Could you check a few things on this model? Use its own coordinates, in mm. A direction names the side the tool comes from. Round coordinates to 2 decimals unless told otherwise and drop trailing zeros. Loops run counter-clockwise (first coordinate to the right, second up) from the corner with the lowest first, then second, coordinate; pieces in that order, holes last. Notation, with made-up numbers: M 28.25,34.5 L 71.25,34.5 A31 ccw 71.25,65.5 Z; hole C 74.5,50.5 d1. An arc over 180 degrees is marked long. Answer in a Markdown table with one row per item.
```python
from build123d import *

# Parameters (mm, degrees)
BOSS_EXTRUDE1_DEPTH = 180.975
FILLET1_R           = 6.35


with BuildPart() as part:
    # Sketch1 → Boss-Extrude1 (new body, symmetric)
    with BuildSketch(Plane(origin=(0, 0, 0), x_dir=(0, 0, -1), z_dir=(1, 0, 0))):
        with BuildLine():
            ThreePointArc((-1.052151583, -0.382951858), (0.017010399, -0.096470768), (1.119676327, 0))
            Line((1.119676327, 0), (138.580323673, 0))
            Line((138.580323673, 0), (138.580323673, 6.35))
            Line((138.580323673, 6.35), (1.119676327, 6.35))
            ThreePointArc((1.119676327, 6.35), (-1.085655529, 6.157058463), (-3.223979493, 5.584096284))
            Line((-3.223979493, 5.584096284), (-72.724254031, -19.711934921))
            Line((-72.724254031, -19.711934921), (-70.552426121, -25.678983063))
            Line((-70.552426121, -25.678983063), (-1.052151583, -0.382951858))
        make_face()
    extrude(amount=BOSS_EXTRUDE1_DEPTH, both=True)

    # Fillet1
    fillet1_edges = [part.edges().sort_by_distance(p)[0] for p in [
        (-180.975, -22.695458992, 71.638340076),
        (180.975, -22.695458992, 71.638340076),
        (180.975, 3.175, -138.580323673),
        (-180.975, 3.175, -138.580323673),
    ]]
    fillet(fillet1_edges, radius=FILLET1_R)


solid = part.part
```
1) I want a section at A-A, the plane x = 95. Please give me the cut outline in (y, z), plus the area to 3 significant figures.
Computed:
| item | result |
|---|---|
| outline | M -25.68,70.55 L -0.38,1.05 A6.35 cw 0,-1.12 L 0,-138.58 L 6.35,-138.58 L 6.35,-1.12 A12.7 ccw 5.58,3.22 L -19.71,72.72 Z |
| area | 1,360 mm² |
2) I want a section at C-C, the plane y = -11. Please give me the cut outline in (x, z) (3 decimals), plus the area to 3 significant figures.
Computed:
| item | result |
|---|---|
| outline | M -180.975,30.222 L 180.975,30.222 L 180.975,48.788 L -180.975,48.788 Z |
| area | 6,720 mm² |
3) I need wall thicknesses on line 1 (Y direction, x = -26.5, z = -65.5); line 2 (Y direction, x = 132, z = 50). Which ranges of each line are inside material? Lowest first, please.
Computed:
| item | result |
|---|---|
| line 1 | y = 0 to 6.35 |
| line 2 | y = -18.2 to -11.44 |
4) I want a section at B-B, the plane z = -58. Please give me the cut outline in (x, y) (3 decimals), plus the area to 3 significant figures.
Computed:
| item | result |
|---|---|
| outline | M -180.975,0 L 180.975,0 L 180.975,6.35 L -180.975,6.35 Z |
| area | 2,300 mm² |
5) Which directions (+Z, -Z, +X, -X, +Y, -Y) give clear straight access to the entire face, cutting with the end or side of a thin tool? Please do faces 1 (the face through (3, 0, -69)), 2 (the face through (180.975, 1, -32)).
Computed:
| item | result |
|---|---|
| face 1 | -Z, +X, -X, -Y |
| face 2 | +Z, -Z, +X, +Y, -Y |
6) Will these pins go through, and if not, where does the flat tip stop? P1, Ø3, axis at x = -26.5, z = 42, coming from the +Y side; P2, Ø5, axis at x = 9.5, z = -51.5, coming from the -Y side; P3, Ø10, axis at x = -14, y = -15.5, coming from the +Z side.
Computed:
| item | result |
|---|---|
| P1 | stops at y = -7.98 |
| P2 | stops at y = 0 |
| P3 | stops at z = 72.72 |
